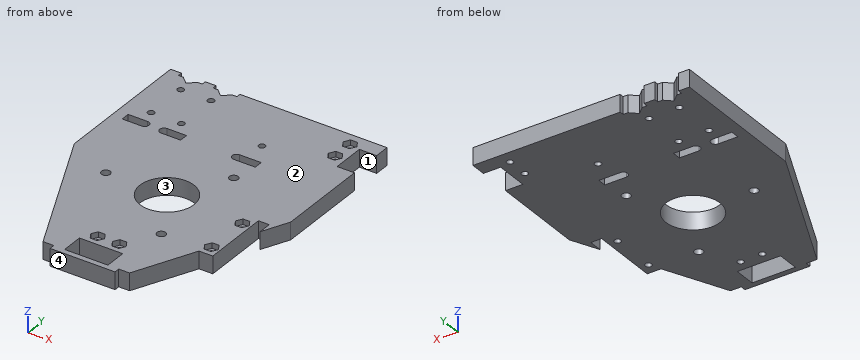
```python
from build123d import *

# Parameters (mm, degrees)
SKETCH_1_W          = 100
SKETCH_1_H          = 130
EXTRUDE_1_DEPTH     = 8
SKETCH_3_W          = 20
SKETCH_3_H          = 10
CUT_EXTRUDE_1_DEPTH = 8
SKETCH_4_R          = 1.5
SKETCH_4_W          = 8
SKETCH_4_H          = 15
CUT_EXTRUDE_2_DEPTH = 9
CUT_EXTRUDE_6_DEPTH = 2.5
SKETCH_10_R         = 12.5
SKETCH_10_W         = 5
SKETCH_10_H         = 30.8
CUT_EXTRUDE_7_DEPTH = 9
EXTRUDE_3_DEPTH     = 8
SKETCH_5_R          = 2
SKETCH_5_R_2        = 1.5
CUT_EXTRUDE_3_DEPTH = 9
SKETCH_11_W         = 30
SKETCH_11_H         = 2.5
EXTRUDE_2_DEPTH     = 8
CUT_EXTRUDE_8_DEPTH = 2.5


with BuildPart() as part:
    # 草图1 → 凸台-拉伸1 (new body)
    with BuildSketch(Plane.XY):
        with Locations((50, 65)):
            Rectangle(SKETCH_1_W, SKETCH_1_H)
    extrude(amount=EXTRUDE_1_DEPTH)

    # 草图3 → 切除-拉伸1 (cut)
    with BuildSketch(Plane.XY.offset(8)):
        with Locations((50, 5)):
            Rectangle(SKETCH_3_W, SKETCH_3_H)
        Polygon((0, 0), (30, 0), (0, 65), align=None)
        Polygon((100, 0), (100, 65), (70, 0), align=None)
    extrude(amount=-CUT_EXTRUDE_1_DEPTH, mode=Mode.SUBTRACT)

    # 草图4 → 切除-拉伸2 (cut, through all)
    with BuildSketch(Plane(origin=(0, 0, 0), x_dir=(-1, 0, 0), z_dir=(0, 0, -1))):
        with Locations((-87, 124)):
            Circle(SKETCH_4_R)
        with Locations((-25.5, 100)):
            Circle(SKETCH_4_R)
        with Locations((-11.5, 100)):
            Circle(SKETCH_4_R)
        with Locations((-11.5, 120)):
            Circle(SKETCH_4_R)
        with Locations((-25.5, 120)):
            Circle(SKETCH_4_R)
        with Locations((-60, 104)):
            Circle(SKETCH_4_R)
        with Locations((-45, 15)):
            Circle(SKETCH_4_R)
        with Locations((-55, 15)):
            Circle(SKETCH_4_R)
        with Locations((-87, 114)):
            Circle(SKETCH_4_R)
        with BuildLine():
            Line((-56.5, 94), (-66.5, 94))
            Line((-66.5, 94), (-66.5, 90))
            Line((-66.5, 90), (-56.5, 90))
            ThreePointArc((-56.5, 90), (-54.5, 92), (-56.5, 94))
        make_face()
        with Locations((-96, 115.5)):
            Rectangle(SKETCH_4_W, SKETCH_4_H)
        with BuildLine():
            Line((-32, 94), (-32, 90))
            Line((-32, 90), (-23, 90))
            ThreePointArc((-23, 90), (-21, 92), (-23, 94))
            Line((-23, 94), (-32, 94))
        make_face()
        with BuildLine():
            Line((-5, 94), (-5, 90))
            Line((-5, 90), (-14, 90))
            ThreePointArc((-14, 90), (-16, 92), (-14, 94))
            Line((-14, 94), (-5, 94))
        make_face()
        Polygon((-10.5, 125), (-13.8, 128), (-16, 128), (-16, 130), (-5, 130), (-5, 128), (-7.2, 128), align=None)
        Polygon((-26.5, 125), (-29.8, 128), (-32, 128), (-32, 130), (-21, 130), (-21, 128), (-23.2, 128), align=None)
    extrude(amount=-CUT_EXTRUDE_2_DEPTH, mode=Mode.SUBTRACT)

    # 草图9 → 切除-拉伸6 (cut)
    with BuildSketch(Plane.XY.offset(8)):
        Polygon((90.175426481, 124), (88.58771324, 126.75), (85.41228676, 126.75), (83.824573519, 124), (85.41228676, 121.25), (88.58771324, 121.25), align=None)
        Polygon((90.175426481, 114), (88.58771324, 116.75), (85.41228676, 116.75), (83.824573519, 114), (85.41228676, 111.25), (88.58771324, 111.25), align=None)
        Polygon((48.175426481, 15), (46.58771324, 17.75), (43.41228676, 17.75), (41.824573519, 15), (43.41228676, 12.25), (46.58771324, 12.25), align=None)
        Polygon((58.175426481, 15), (56.58771324, 17.75), (53.41228676, 17.75), (51.824573519, 15), (53.41228676, 12.25), (56.58771324, 12.25), align=None)
    extrude(amount=-CUT_EXTRUDE_6_DEPTH, mode=Mode.SUBTRACT)

    # 草图10 → 切除-拉伸7 (cut, through all)
    with BuildSketch(Plane.XY.offset(8)):
        with Locations((50, 54.5)):
            Circle(SKETCH_10_R)
        with Locations((91.8, 43.4)):
            Rectangle(SKETCH_10_W, SKETCH_10_H)
    extrude(amount=-CUT_EXTRUDE_7_DEPTH, mode=Mode.SUBTRACT)

    # 草图12 → 凸台-拉伸3 (add)
    with BuildSketch(Plane.XY.offset(8)):
        Polygon((89.3, 41.816666667), (82.923076923, 28), (89.3, 28), align=None)
    extrude(amount=-EXTRUDE_3_DEPTH)

    # 草图5 → 切除-拉伸3 (cut, through all)
    with BuildSketch(Plane.XY.offset(8)):
        with Locations((21.75, 54.5)):
            Circle(SKETCH_5_R)
        with Locations((64.125, 78.965217657)):
            Circle(SKETCH_5_R)
        with Locations((64.125, 30.034782343)):
            Circle(SKETCH_5_R)
        with Locations((85.3, 53.8)):
            Circle(SKETCH_5_R_2)
        with Locations((85.3, 33)):
            Circle(SKETCH_5_R_2)
    extrude(amount=-CUT_EXTRUDE_3_DEPTH, mode=Mode.SUBTRACT)

    # 草图11 → 凸台-拉伸2 (add)
    with BuildSketch(Plane.XY.offset(8)):
        with Locations((50, -1.25)):
            Rectangle(SKETCH_11_W, SKETCH_11_H)
    extrude(amount=-EXTRUDE_2_DEPTH)

    # 草图14 → 切除-拉伸8 (cut)
    with BuildSketch(Plane.XY.offset(8)):
        Polygon((88.475426481, 53.8), (86.88771324, 56.55), (83.71228676, 56.55), (82.124573519, 53.8), (83.71228676, 51.05), (86.88771324, 51.05), align=None)
        Polygon((88.475426481, 33), (86.88771324, 35.75), (83.71228676, 35.75), (82.124573519, 33), (83.71228676, 30.25), (86.88771324, 30.25), align=None)
    extrude(amount=-CUT_EXTRUDE_8_DEPTH, mode=Mode.SUBTRACT)


solid = part.part
```
For this review, take the finished solid that the model builds, in its own axes (mm). Face numbers are marked on the shaded views. Give positions to 0.01 mm unless a question says otherwise; leave off trailing zeros. Write each loop counter-clockwise with the first axis right and the second up, starting at its lowest first coordinate (ties: lowest second). Pieces come first, ordered by that corner, then holes.
Item 1: Take a section at B-B (x = 45). Give the boundary of the cut face in (y, z), and give its area (3 significant figures).
Item 2: Wall thickness on probe 1 along Y at (x, z) = (85.3, 1.3); probe 2 along Y at (x, z) = (11.5, 3.75); probe 3 along Y at (x, z) = (55, 1.25): over which ranges is each line inside the solid? List them lowest first.
Item 3: Insertion check: P1, Ø1.6, axis at x = 46.5, y = 15.5, coming from the +Z side; P2, Ø1.5, axis at x = 15, z = 1.5, coming from the -Y side (3 decimals); P3, Ø1.1, axis at x = 22.5, z = 2.5, coming from the +Y side. Each pin has a flat end and moves straight along its axis. Give the tip position at first contact, or say it passes through.
Item 4: The part is to be moulded in two halves that separate along Y. For the marked faces 1, 2, 3 and 4, say which applies: +Y half, -Y half, draft (parallel to the pull), parting line (faces both ways), or undercut.
Item 5: Take a section at A-A (y = 92). Give the boundary of the cut face in (x, z), and give its area (3 significant figures).
Established:
1. outline: (-2.5, 0) - (0, 0) - (0, 8) - (-2.5, 8) - close; (10, 0) - (13.5, 0) - (13.5, 5.5) - (12.25, 5.5) - (12.25, 8) - (10, 8) - close; (16.5, 0) - (43.04, 0) - (43.04, 8) - (17.75, 8) - (17.75, 5.5) - (16.5, 5.5) - close; (65.96, 0) - (130, 0) - (130, 8) - (65.96, 8) - close
1. area: 766 mm2
2. probe 1: y = 28 to 31.5, 34.5 to 52.3, 55.3 to 130
2. probe 2: y = 40.08 to 90, 94 to 98.5, 101.5 to 118.5, 121.5 to 125.91
2. probe 3: y = -2.5 to 0, 10 to 13.5, 16.5 to 43.04, 65.96 to 90.68, 93.32 to 130
3. P1: stops at z = 5.5
3. P2: stops at y = 30.875
3. P3: stops at y = 128
4. face 1: undercut
4. face 2: draft
4. face 3: undercut
4. face 4: -Y half
5. outline: (0, 0) - (5, 0) - (5, 8) - (0, 8) - close; (16, 0) - (21, 0) - (21, 8) - (16, 8) - close; (32, 0) - (54.5, 0) - (54.5, 8) - (32, 8) - close; (66.5, 0) - (100, 0) - (100, 8) - (66.5, 8) - close
5. area: 528 mm2
